Model file for the job. Use its own axes, mm. A direction names the side the tool comes from. Round coordinates to 2 decimals unless told otherwise and drop trailing zeros. Loops run counter-clockwise (first coordinate to the right, second up) from the corner with the lowest first, then second, coordinate; pieces in that order, holes last. Notation, with made-up numbers: (-20.5, 48.25) - (-10.5, 48.25) arc R9 cw to (-10.5, 59.25) - close; hole circle Ø6 at (54.25, 41). An arc over 180 degrees is marked (long way). Answer as a JSON object with one key per item and string values.
from build123d import *

# Parameters (mm, degrees)
F0_R     = 3
F0_R_2   = 2
F1_DEPTH = 3
F2_DEPTH = 53
F3_DEPTH = 33


with BuildPart() as f1:
    # F0 (on Top) → F1 (new body)
    with BuildSketch(Plane.XY):
        Polygon((-11.9926406871, 10.25), (-22.2426406871, 0), (-11.9926406871, -10.25), (11.9926406871, -10.25), (22.2426406871, 0), (11.9926406871, 10.25), align=None)
        Polygon((-18, 0), (-10.75, 7.25), (10.75, 7.25), (18, 0), (10.75, -7.25), (-10.75, -7.25), align=None, mode=Mode.SUBTRACT)
        Polygon((10.75, 7.25), (-10.75, 7.25), (-18, 0), (-10.75, -7.25), (10.75, -7.25), (18, 0), align=None)
        with Locations((-9.5, 0)):
            Circle(F0_R, mode=Mode.SUBTRACT)
        with Locations((9.5, 0)):
            Circle(F0_R, mode=Mode.SUBTRACT)
        Polygon((32.2426406871, 10.25), (11.9926406871, 10.25), (22.2426406871, 0), (11.9926406871, -10.25), (32.2426406871, -10.25), align=None)
        with Locations((27.2426406871, 0)):
            Circle(F0_R_2, mode=Mode.SUBTRACT)
        Polygon((-11.9926406871, -10.25), (-22.2426406871, 0), (-11.9926406871, 10.25), (-32.2426406871, 10.25), (-32.2426406871, -10.25), align=None)
        with Locations((-27.2426406871, 0)):
            Circle(F0_R_2, mode=Mode.SUBTRACT)
        with Locations((-9.5, 0)):
            Circle(F0_R)
        with Locations((9.5, 0)):
            Circle(F0_R)
    extrude(amount=F1_DEPTH)

    # F0 (on Top) → F2 (join)
    with BuildSketch(Plane.XY):
        Polygon((-11.9926406871, 10.25), (-22.2426406871, 0), (-11.9926406871, -10.25), (11.9926406871, -10.25), (22.2426406871, 0), (11.9926406871, 10.25), align=None)
        Polygon((-18, 0), (-10.75, 7.25), (10.75, 7.25), (18, 0), (10.75, -7.25), (-10.75, -7.25), align=None, mode=Mode.SUBTRACT)
    extrude(amount=F2_DEPTH)

    # F0 (on Top) → F3 (join)
    with BuildSketch(Plane.XY):
        Polygon((10.75, 7.25), (-10.75, 7.25), (-18, 0), (-10.75, -7.25), (10.75, -7.25), (18, 0), align=None)
        with Locations((-9.5, 0)):
            Circle(F0_R, mode=Mode.SUBTRACT)
        with Locations((9.5, 0)):
            Circle(F0_R, mode=Mode.SUBTRACT)
    extrude(amount=F3_DEPTH)


solid = f1.part
1) Slice it at D-D on x = -1.5. List the corners of the cut face in (y, z).
Values follow:
{"outline": "(-10.25, 0) - (10.25, 0) - (10.25, 53) - (7.25, 53) - (7.25, 33) - (-7.25, 33) - (-7.25, 53) - (-10.25, 53) - close"}
2) Slice it at A-A on z = 7. List the corners of the cut face in (x, y).
Values follow:
{"outline": "(-22.24, 0) - (-11.99, -10.25) - (11.99, -10.25) - (22.24, 0) - (11.99, 10.25) - (-11.99, 10.25) - close; hole circle Ø6 at (-9.5, 0); hole circle Ø6 at (9.5, 0)"}
3) Slice it at B-B on z = 36. List the corners of the cut face in (x, y).
Values follow:
{"outline": "(-22.24, 0) - (-11.99, -10.25) - (11.99, -10.25) - (22.24, 0) - (11.99, 10.25) - (-11.99, 10.25) - close; hole (-18, 0) - (-10.75, -7.25) - (10.75, -7.25) - (18, 0) - (10.75, 7.25) - (-10.75, 7.25) - close"}
4) Slice it at C-C on y = -1. List the corners of the cut face in (x, z), then the cut area to 3 significant figures.
Values follow:
{"outline": "(-32.24, 0) - (-28.97, 0) - (-28.97, 3) - (-32.24, 3) - close; (-25.51, 0) - (25.51, 0) - (25.51, 3) - (21.24, 3) - (21.24, 53) - (17, 53) - (17, 33) - (12.33, 33) - (12.33, 3) - (6.67, 3) - (6.67, 33) - (-6.67, 33) - (-6.67, 3) - (-12.33, 3) - (-12.33, 33) - (-17, 33) - (-17, 53) - (-21.24, 53) - (-21.24, 3) - (-25.51, 3) - close; (28.97, 0) - (32.24, 0) - (32.24, 3) - (28.97, 3) - close", "area": "1,280 mm²"}
5) Two-plate mould, pull along X, no slides. Class faces 6 (the flat face through (-17.19, -5.05, 27.65)), 7 (the flat face through (24, 0, 3)), 8 (the flat face through (17.19, 5.05, 27.65)), 9 (the flat face through (0, 7.25, 43)): pulls with the +X half, pulls with the -X half, needs draft (parallel to the pull), parting line crosses it, or undercut.
Values follow:
{"face 6": "pulls with the -X half", "face 7": "needs draft", "face 8": "pulls with the +X half", "face 9": "undercut"}
6) Probe probe 1 along X at (y, z) = (0, 21.5); probe 2 along Y at (x, z) = (-3.5, 41); probe 3 along Z at (x, y) = (14, 3.25). List the from-to ranges inside material, lowest first.
Values follow:
{"probe 1": "-22.24 to -12.5, -6.5 to 6.5, 12.5 to 22.24", "probe 2": "-10.25 to -7.25, 7.25 to 10.25", "probe 3": "0 to 33"}
7) Tool access for faces 1 (the flat face through (17.046, -5.197, 27.65)), 2 (the flat face through (-32.243, 0, 1)), 3 (the flat face through (9, 0, 3)), 4 (the cylindrical face through (-25.335, 0.601, 1.479)), 5 (the flat face through (-17.046, 5.197, 27.65)): list every direction of +Z, -Z, +X, -X, +Y, -Y with a clear straight run to the whole face (end or side of a thin tool).
Values follow:
{"face 1": "+Z, +X, -Y", "face 2": "+Z, -Z, -X, +Y, -Y", "face 3": "+Z", "face 4": "+Z, -Z", "face 5": "+Z, -X, +Y"}
8) Drop flat-ended pins along their axis: P1, Ø6, axis at x = 19, z = 15, coming from the -Y side; P2, Ø8, axis at x = 3.5, y = -2.5, coming from the +Z side; P3, Ø10, axis at x = 26.5, y = -3.5, coming from the +Z side. Give the stop position or say it passes through.
Values follow:
{"P1": "y = -6.24", "P2": "z = 33", "P3": "z = 3"}
